from build123d import *

# Parameters (mm, degrees)
SKETCH2_W          = 25
SKETCH2_H          = 25
SKETCH2_W_2        = 22.2
SKETCH2_H_2        = 22.2
CUT_EXTRUDE1_REACH = 192.87
SKETCH3_R          = 5


with BuildPart() as part:
    # Sweep1: sweep along a path in Sketch1
    with BuildLine(Plane(origin=(0, 0, 0), x_dir=(1, 0, 0), z_dir=(0, 1, 0))) as sweep1_path:
        Line((-125, -130), (-125, 0))
        Line((-125, 0), (125, 0))
        Line((125, 0), (125, -130))
    # Sketch2 → Sweep1 (sweep)
    with BuildSketch(Plane(origin=(-125, 0, 130), x_dir=(-1, 0, 0), z_dir=(0, 0, -1))):
        Rectangle(SKETCH2_W, SKETCH2_H)
        Rectangle(SKETCH2_W_2, SKETCH2_H_2, mode=Mode.SUBTRACT)
    sweep(path=sweep1_path.line, transition=Transition.RIGHT)

    # Cut-Extrude1: up to this face of the body (flat: up to its plane)
    cut_extrude1_end = Plane(part.part.faces().sort_by_distance((-115.59727703, -12.5, 71.25))[0])
    # Sketch3 → Cut-Extrude1 (cut, up to the picked face)
    with BuildSketch(Plane(origin=(0, 12.5, 0), x_dir=(1, 0, 0), z_dir=(0, 1, 0)), mode=Mode.PRIVATE) as cut_extrude1_sk1:
        with Locations(Location((77.5, 0, 0), (0, 0, 270))):
            Circle(SKETCH3_R)
    cut_extrude1_tool1 = split(extrude(cut_extrude1_sk1.sketch, amount=-CUT_EXTRUDE1_REACH, mode=Mode.PRIVATE), bisect_by=cut_extrude1_end, keep=Keep.BOTH, mode=Mode.PRIVATE)
    # Sketch3 → Cut-Extrude1 (cut, up to the picked face)
    with BuildSketch(Plane(origin=(0, 12.5, 0), x_dir=(1, 0, 0), z_dir=(0, 1, 0)), mode=Mode.PRIVATE) as cut_extrude1_sk2:
        with Locations(Location((-107.5, 0, 0), (0, 0, 270))):
            Circle(SKETCH3_R)
    cut_extrude1_tool2 = split(extrude(cut_extrude1_sk2.sketch, amount=-CUT_EXTRUDE1_REACH, mode=Mode.PRIVATE), bisect_by=cut_extrude1_end, keep=Keep.BOTH, mode=Mode.PRIVATE)
    add(cut_extrude1_tool1.solids().sort_by(Axis((77.5, 12.5, 0), (0, -1, 0)))[0], mode=Mode.SUBTRACT)
    add(cut_extrude1_tool2.solids().sort_by(Axis((-107.5, 12.5, 0), (0, -1, 0)))[0], mode=Mode.SUBTRACT)


solid = part.part
Can you work these out from the model? Positions are in its coordinate system, mm. A direction names the side the tool comes from. Give positions to 0.01 mm unless a question says otherwise; leave off trailing zeros. Loops run counter-clockwise (first coordinate to the right, second up) from the corner with the lowest first, then second, coordinate; pieces in that order, holes last. Notation, with made-up numbers: (19.25, -22.5) - (77.25, -22.5) arc R7 cw to (77.25, -13.5) - close; hole circle Ø5 at (50.5, -0.75). An arc over 180 degrees is marked (long way). Answer as a JSON object with one key per item and string values.
Q1. Which directions (+Z, -Z, +X, -X, +Y, -Y) give clear straight access to the entire face, cutting with the end or side of a thin tool? Please do faces 4 (the flat face through (2, 0, 12.5)), 5 (the flat face through (9, -11.1, 7)), 6 (the flat face through (-136.1, 0, 58)).
Geometry says:
{"face 4": "+Z, +Y, -Y", "face 5": "none", "face 6": "+Z"}
Q2. If we mould it in two halves opening along Z, with no side actions, what happens to faces 1 (the cylindrical face through (72.62, 11.81, -1.08)), 2 (the flat face through (136.1, 0, 60)), 3 (the flat face through (2, 0, -12.5))? For each: pulls with the +Z half, pulls with the -Z half, needs draft (parallel to the pull), parting line crosses it, or undercut.
Geometry says:
{"face 1": "undercut", "face 2": "needs draft", "face 3": "pulls with the -Z half"}
Q3. Will these pins go through, and if not, where does the flat tip stop? P1, Ø5, axis at x = -53.5, y = 5, coming from the +Z side; P2, Ø6, axis at x = 77.5, z = 0, coming from the +Y side.
Geometry says:
{"P1": "z = 12.5", "P2": "through"}
Q4. If I drill on L1, parallel to X at y = -12.1, z = 0; L2, parallel to X at y = 5.75, z = 122.5; L3, parallel to Y at x = 120.5, z = 37, over which ranges is the centre line in solid material (lowest first)?
Geometry says:
{"L1": "-137.5 to -112.5, -102.5 to 72.5, 82.5 to 137.5", "L2": "-137.5 to -136.1, -113.9 to -112.5, 112.5 to 113.9, 136.1 to 137.5", "L3": "-12.5 to -11.1, 11.1 to 12.5"}
Q5. Imagine slicing it at D-D on x = 77.5. Write out the boundary of the cut face in (y, z), plus the area to 3 significant figures.
Geometry says:
{"outline": "(-12.5, -12.5) - (12.5, -12.5) - (12.5, -5) - (11.1, -5) - (11.1, -11.1) - (-11.1, -11.1) - (-11.1, -5) - (-12.5, -5) - close; (-12.5, 5) - (-11.1, 5) - (-11.1, 11.1) - (11.1, 11.1) - (11.1, 5) - (12.5, 5) - (12.5, 12.5) - (-12.5, 12.5) - close", "area": "104 mm²"}
Q6. Imagine slicing it at A-A on z = 0. Write out the boundary of the cut face in (x, y).
Geometry says:
{"outline": "(-137.5, -12.5) - (-112.5, -12.5) - (-112.5, -11.1) - (-136.1, -11.1) - (-136.1, 11.1) - (-112.5, 11.1) - (-112.5, 12.5) - (-137.5, 12.5) - close; (-102.5, -12.5) - (72.5, -12.5) - (72.5, -11.1) - (-102.5, -11.1) - close; (-102.5, 11.1) - (72.5, 11.1) - (72.5, 12.5) - (-102.5, 12.5) - close; (82.5, -12.5) - (137.5, -12.5) - (137.5, 12.5) - (82.5, 12.5) - (82.5, 11.1) - (136.1, 11.1) - (136.1, -11.1) - (82.5, -11.1) - close"}
Q7. Imagine slicing it at C-C on z = 121. Write out the boundary of the cut face in (x, y).
Geometry says:
{"outline": "(-137.5, -12.5) - (-112.5, -12.5) - (-112.5, 12.5) - (-137.5, 12.5) - close; (112.5, -12.5) - (137.5, -12.5) - (137.5, 12.5) - (112.5, 12.5) - close; hole (-136.1, -11.1) - (-113.9, -11.1) - (-113.9, 11.1) - (-136.1, 11.1) - close; hole (113.9, -11.1) - (136.1, -11.1) - (136.1, 11.1) - (113.9, 11.1) - close"}
Q8. Imagine slicing it at B-B on y = -5. Write out the boundary of the cut face in (x, z).
Geometry says:
{"outline": "(-137.5, -12.5) - (137.5, -12.5) - (137.5, 130) - (136.1, 130) - (136.1, -11.1) - (-136.1, -11.1) - (-136.1, 130) - (-137.5, 130) - close; (-113.9, 11.1) - (113.9, 11.1) - (113.9, 130) - (112.5, 130) - (112.5, 12.5) - (-112.5, 12.5) - (-112.5, 130) - (-113.9, 130) - close"}
